Part model, mm, in its own coordinate system. Face numbers are marked on the shaded views. A direction names the side the tool comes from. Coordinates: 2 decimals unless noted, no trailing zeros. Order: outer loops, then holes, each group sorted by start corner. A loop starts at its lowest first (then second) coordinate and runs counter-clockwise, first axis right, second up.
1) Cut at C-C (y = 5.25). List the corners of the cut face in (x, z).
2) Tool access for the marked faces 1 and 2: list every direction of +Z, -Z, +X, -X, +Y, -Y with a clear straight run to the whole face (end or side of a thin tool).
3) Pin check, flat tips, straight feed: pin 1 Ø10 at (x, y) = (9.5, 2.5) entering from +Z; pin 2 Ø2 at (y, z) = (5.5, 2) entering from +X; pin 3 Ø6 at (x, y) = (0, 0) entering from +Z; pin 4 Ø3 at (y, z) = (9.5, 5) entering from +X. Stop position of each tip, or through.
4) Wall check: L1, parallel to Y at x = 0, z = 3; L2, parallel to Y at x = 33.5, z = 5.5; L3, parallel to Y at x = -1.5, z = 0.5. Give the ranges that are in metal, low to high.
5) Cut at A-A (x = 0). List the corners of the cut face in (y, z).
6) Cut at B-B (z = 5). List the corners of the cut face in (x, y), and give its area (3 significant figures).
7) Cut at D-D (z = 12). List the corners of the cut face in (x, y), and give its area (3 significant figures).
8) Mould opens along X. For the marked faces 3, 4, 5 and 6 say: +X half, -X half, draft (parallel to the pull), parting line (faces both ways), or undercut.
```python
from build123d import *

# Parameters (mm, degrees)
SKETCH_1_R      = 3.4
EXTRUDE_1_DEPTH = 7
SKETCH_2_W      = 50
SKETCH_2_H      = 15
EXTRUDE_2_DEPTH = 3


with BuildPart() as part:
    # 草图1 → 凸台-拉伸1 (new body)
    with BuildSketch(Plane.XY):
        with BuildLine():
            Line((-5, 0), (-5, 10))
            Line((-5, 10), (5, 10))
            Line((5, 10), (5, 0))
            ThreePointArc((5, 0), (0, -5), (-5, 0))
        make_face()
        Circle(SKETCH_1_R, mode=Mode.SUBTRACT)
    extrude(amount=EXTRUDE_1_DEPTH)

    # 草图2 → 凸台-拉伸2 (add)
    with BuildSketch(Plane(origin=(0, 10, 0), x_dir=(1, 0, 0), z_dir=(0, 1, 0))):
        with Locations((20, -7.5)):
            Rectangle(SKETCH_2_W, SKETCH_2_H)
    extrude(amount=EXTRUDE_2_DEPTH)


solid = part.part
```
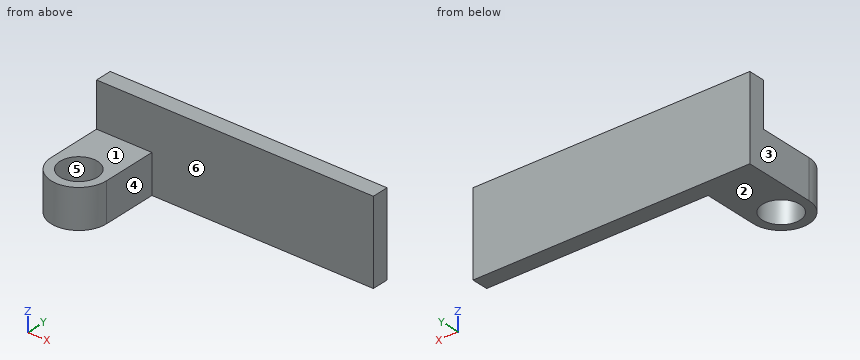
Geometry check:
1. outline: (-5, 0) - (5, 0) - (5, 7) - (-5, 7) - close
2. face 1: +Z, +X, -X, -Y
2. face 2: -Z, +X, -X, +Y, -Y
3. pin 1: stops at z = 7
3. pin 2: stops at x = 5
3. pin 3: passes through
3. pin 4: stops at x = 45
4. L1: y = -5 to -3.4, 3.4 to 13
4. L2: y = 10 to 13
4. L3: y = -4.77 to -3.05, 3.05 to 13
5. outline: (-5, 0) - (-3.4, 0) - (-3.4, 7) - (-5, 7) - close; (3.4, 0) - (13, 0) - (13, 15) - (10, 15) - (10, 7) - (3.4, 7) - close
6. outline: (-5, 0) arc R5 ccw to (5, 0) - (5, 10) - (45, 10) - (45, 13) - (-5, 13) - close; hole circle Ø6.8 at (0, 0)
6. area: 253 mm2
7. outline: (-5, 10) - (45, 10) - (45, 13) - (-5, 13) - close
7. area: 150 mm2
8. face 3: -X half
8. face 4: +X half
8. face 5: undercut
8. face 6: draft
